Autodesk Inventor part; units mm, degrees
ref_plane "YZ Plane" through (0, 0, 0) normal (1, 0, 0) x (0, 1, 0)
ref_plane "XZ Plane" through (0, 0, 0) normal (0, 1, 0) x (-1, 0, 0)
ref_plane "XY Plane" through (0, 0, 0) normal (0, 0, 1) x (1, 0, 0)
sketch "Sketch1" plane through (0, 0, 0) normal (0, 1, 0) x (-1, 0, 0)
  line L0 (-21.4, -21.65) -> (21.4, -21.65)
  line L1 (21.4, -21.65) -> (21.4, 21.65)
  line L2 (21.4, 21.65) -> (-21.4, 21.65)
  line L3 (-21.4, 21.65) -> (-21.4, -21.65)
  line L4 (-21.4, -21.65) -> (21.4, 21.65) construction
  line L5 (21.4, -21.65) -> (-21.4, 21.65) construction
  point P0 (0, 0)
  dimension "d0" = 43.3
  dimension "d1" = 42.8
extrude "Extrusion1" add sketch "Sketch1" along normal blind 1.5
sketch "Sketch2" plane through (0, 1.5, 0) normal (0, 1, 0) x (1, 0, 0)
  line L0 (22.9, 23.15) -> (-22.9, 23.15)
  line L1 (-22.9, 23.15) -> (-22.9, -23.15)
  line L2 (-22.9, -23.15) -> (22.9, -23.15)
  line L3 (22.9, -23.15) -> (22.9, 23.15)
  line L4 (22.9, 23.15) -> (-22.9, -23.15) construction
  line L5 (-22.9, 23.15) -> (22.9, -23.15) construction
  line L6 (-21.4, 21.65) -> (-21.4, -21.65)
  line L7 (-21.4, -21.65) -> (21.4, -21.65)
  point P0 (0, 0)
  dimension "d4" = 1.5
  dimension "d5" = 1.5
extrude "Extrusion2" add sketch "Sketch2" along normal blind 1.5
sketch "Sketch3" plane through (0, 3, 0) normal (0, 1, 0) x (1, 0, 0)
  line L0 (19.9, 20.15) -> (-19.9, 20.15)
  line L1 (-19.9, 20.15) -> (-19.9, -20.15)
  line L2 (-19.9, -20.15) -> (19.9, -20.15)
  line L3 (19.9, -20.15) -> (19.9, 20.15)
  line L4 (19.9, 20.15) -> (-19.9, -20.15) construction
  line L5 (-19.9, 20.15) -> (19.9, -20.15) construction
  line L6 (-21.4, -21.65) -> (21.4, -21.65)
  line L7 (-21.4, 21.65) -> (-21.4, -21.65)
  point P0 (0, 0)
  dimension "d8" = 1.5
  dimension "d9" = 1.5
extrude "Extrusion3" cut sketch "Sketch3" against normal through all
chamfer "Chamfer1" distance 2.9 angle 45 2 edges at (22.9, 2.25, -23.15) (-22.9, 2.25, 23.15)
sketch "Sketch4" plane through (21.4, 0, 21.65) normal (1, 0, 0) x (0, 0, -1)
  line L0 (1.4, 1.5) -> (-1.5, 1.5)
  line L1 (-0.75, 1.5) -> (44.05, 1.5)
  line L2 (44.05, 1.5) -> (44.05, 0)
  line L3 (44.05, 0) -> (-0.75, 0)
  line L4 (-0.75, 0) -> (-0.75, 1.5)
  line L5 (0, 0) -> (43.3, 0)
  line L6 (-0.75, 0.75) -> (0, 0)
  line L7 (-0.75, 0.75) -> (0, 1.5)
  line L8 (21.65, 9.7528) -> (21.65, -18.8519)
  line L9 (0, 0) -> (0, 1.5)
  line L10 (44.05, 0.75) -> (43.3, 0)
  line L11 (44.05, 0.75) -> (43.3, 1.5)
  line L12 (43.3, 0) -> (43.3, 1.5)
  point P0 (21.65, 0)
  point P1 (21.65, 0)
  point P2 (21.65, 0)
  dimension "d16" = 44.8
  dimension "d17" = 22.4
  dimension "d18" = 0.75
extrude "Extrusion4" add sketch "Sketch4" against normal up to surface (42.8 mm away) contours L9 L6 L7 | L11 L10 L12
chamfer "Chamfer2" distance 0.5 angle 45 8 edges at (-21.4, 0.375, -22.025) (-21.4, 1.125, -22.025) (-21.4, 0.375, 22.025) (-21.4, 1.125, 22.025) (21.4, 0.375, 22.025) (21.4, 1.125, 22.025) (21.4, 0.375, -22.025) (21.4, 1.125, -22.025)
properties part number "Installation Tool Collar"
For this review, take the finished solid that the model builds, in its own axes (mm). A direction names the side the tool comes from. Round coordinates to 2 decimals unless told otherwise and drop trailing zeros. Write each loop counter-clockwise with the first axis right and the second up, starting at its lowest first coordinate (ties: lowest second). Pieces come first, ordered by that corner, then holes. Notation, with made-up numbers: (-14, 40.25) - (33, 40.25) arc R31 ccw to (33, 66.25) - close; hole circle Ø10 at (86.25, -31). An arc over 180 degrees is marked (long way). Put each result on its own line as item: value.
Q1. Machinability: for faces 1 (the face through (19.9, 2, 0)), 2 (the face through (-21.4, 1, 0)), 3 (the face through (-22, 1.5, 0)), 4 (the face through (21.4, 1, 0)), which of the approach directions +Z, -Z, +X, -X, +Y, -Y give a long, thin tool a straight path to every point of the face, cutting with its end or side? Answer none if there is none.
Solved:
face 1: +Y, -Y
face 2: +Z, -Z, -X, -Y
face 3: none
face 4: +Z, -Z, +X, -Y
Q2. Mouldability with a two-part tool opening along X and no side actions: class faces 5 (the face through (21.43, 2.26, -21.72)), 6 (the face through (-19.9, 2, 0)), 7 (the face through (1, 2, 23.15)), 8 (the face through (-21.47, 2.24, 21.68)) as released by +X, released by -X, zero draft, split by the parting line, or undercut.
Solved:
face 5: released by +X
face 6: undercut
face 7: zero draft
face 8: released by -X
Q3. We need section A-A (z = 2). Give the boundary of the cut face in (x, y).
Solved:
outline: (-22.9, 1.5) - (-21.4, 1.5) - (-21.4, 0) - (-19.9, 0) - (-19.9, 3) - (-22.9, 3) - close; (19.9, 0) - (21.4, 0) - (21.4, 1.5) - (22.9, 1.5) - (22.9, 3) - (19.9, 3) - close
Q4. We need section B-B (x = 0.5). Give the boundary of the cut face in (y, z).
Solved:
outline: (0, -21.65) - (0.75, -22.4) - (1.5, -21.65) - (1.5, -23.15) - (3, -23.15) - (3, -20.15) - (0, -20.15) - close; (0, 20.15) - (3, 20.15) - (3, 23.15) - (1.5, 23.15) - (1.5, 21.65) - (0.75, 22.4) - (0, 21.65) - close
Q5. We need section C-C (y = 2.4). Give the boundary of the cut face in (x, z), and give its area (3 significant figures).
Solved:
outline: (-22.9, -23.15) - (20, -23.15) - (22.9, -20.25) - (22.9, 23.15) - (-20, 23.15) - (-22.9, 20.25) - close; hole (-19.9, -20.15) - (19.9, -20.15) - (19.9, 20.15) - (-19.9, 20.15) - close
area: 508 mm2
Q6. Wall thickness on probe 1 along X at (y, z) = (2, -14.5); probe 2 along X at (y, z) = (1.1, -8); probe 3 along Z at (x, y) = (2, 2.25): over which ranges is each line inside the solid? List them lowest first.
Solved:
probe 1: x = -22.9 to -19.9, 19.9 to 22.9
probe 2: x = -21.4 to -19.9, 19.9 to 21.4
probe 3: z = -23.15 to -20.15, 20.15 to 23.15
Q7. Insertion check: pin 1 Ø10 at (x, z) = (-17, 3) entering from +Y; pin 2 Ø0.8 at (y, z) = (0.5, -1.5) entering from -X; pin 3 Ø0.5 at (y, z) = (1, -7.5) entering from +X. Each pin has a flat end and moves straight along its axis. Give the tip position at first contact, or say it passes through.
Solved:
pin 1: stops at y = 3
pin 2: stops at x = -21.4
pin 3: stops at x = 21.4
